Input: part model. Units: mm. Frame: model coordinates. A direction names the side the tool comes from. Round coordinates to 2 decimals unless told otherwise and drop trailing zeros. Order: outer loops, then holes, each group sorted by start corner. A loop starts at its lowest first (then second) coordinate and runs counter-clockwise, first axis right, second up. Notation, with made-up numbers: (45, 71.5) -> (103, 71.5) arc R24 ccw to (103, 92.5) -> close; hole circle Ø8 at (-37.75, 38). An arc over 180 degrees is marked (long way). Use a Markdown table: item, result.
from build123d import *

# Parameters (mm, degrees)
F0_R     = 3.175
F1_DEPTH = 38.1
F3_DEPTH = 2.54


with BuildPart() as f1:
    # F0 (on Front) → F1 (new body)
    with BuildSketch(Plane.XZ):
        Circle(F0_R)
    extrude(amount=-F1_DEPTH)

    # F2 (on face) → F3 (join)
    with BuildSketch(Plane.XZ):
        with BuildLine():
            Line((-6.35, 0), (-19.05, 0))
            ThreePointArc((-19.05, 0), (0, -19.05), (19.05, 0))
            Line((19.05, 0), (6.35, 0))
            Line((6.35, 0), (6.35, 38.1))
            Line((6.35, 38.1), (-6.35, 38.1))
            Line((-6.35, 38.1), (-6.35, 0))
        make_face()
    extrude(amount=F3_DEPTH)


solid = f1.part
1) Pin query (flat end, axial travel): pin 1 Ø6 at (x, z) = (5, 11) entering from +Y; pin 2 Ø2 at (y, z) = (-2, 14) entering from -X; pin 3 Ø3 at (x, y) = (6, 16) entering from +Z; pin 4 Ø2 at (y, z) = (-1, 17) entering from +X. Return the tip coordinate at first contact, or that it passes through.
Results found:
| item | result |
|---|---|
| pin 1 | stops at y = 0 |
| pin 2 | stops at x = -6.35 |
| pin 3 | passes through |
| pin 4 | stops at x = 6.35 |
2) Cut plane D-D on z = -4.5. Return loops of the section in (x, y), and give its area (3 significant figures).
Results found:
| item | result |
|---|---|
| outline | (-18.51, -2.54) -> (18.51, -2.54) -> (18.51, 0) -> (-18.51, 0) -> close |
| area | 94.0 mm² |
3) Cut plane C-C on y = 20. Return loops of the section in (x, z) (3 decimals).
Results found:
| item | result |
|---|---|
| outline | circle Ø6.35 at (0, 0) |
4) Cut plane A-A on x = 0. Return loops of the section in (y, z) (3 decimals).
Results found:
| item | result |
|---|---|
| outline | (-2.54, -19.05) -> (0, -19.05) -> (0, -3.175) -> (38.1, -3.175) -> (38.1, 3.175) -> (0, 3.175) -> (0, 38.1) -> (-2.54, 38.1) -> close |
5) Line query: L1, parallel to Y at x = -5.5, z = 18.5; L2, parallel to Z at x = 2.5, y = 30; L3, parallel to Z at x = -0.5, y = 13.5. Output: solid intervals per line, ascending. Write a range as [from, to].
Results found:
| item | result |
|---|---|
| L1 | y = [-2.54, 0] |
| L2 | z = [-1.96, 1.96] |
| L3 | z = [-3.14, 3.14] |
6) Set-up query: faces 1 (the cylindrical face through (-0.69, 18.78, -3.1)), 2 (the flat face through (0, -1, 38.1)), 3 (the cylindrical face through (-0.419, -1.252, -19.045)), 4 (the flat face through (-6.35, -1, 19)), 5 (the flat face through (6.35, -1, 19)). Return all of +Z, -Z, +X, -X, +Y, -Y with unobstructed straight access to the full face (end or side cutting, diameter ignored); none if empty.
Results found:
| item | result |
|---|---|
| face 1 | +Y |
| face 2 | +Z, +X, -X, +Y, -Y |
| face 3 | -Z, +Y, -Y |
| face 4 | +Z, -X, +Y, -Y |
| face 5 | +Z, +X, +Y, -Y |
7) Cut plane B-B on z = 31.5. Return loops of the section in (x, y), and give its area (3 significant figures).
Results found:
| item | result |
|---|---|
| outline | (-6.35, -2.54) -> (6.35, -2.54) -> (6.35, 0) -> (-6.35, 0) -> close |
| area | 32.3 mm² |
